For this review, use the dimensioned drawing (mm, ordinates from the lowest corner) and the shaded views. Give positions to 0.01 mm unless a question says otherwise; leave off trailing zeros. Order: outer loops, then holes, each group sorted by start corner. A loop starts at its lowest first (then second) coordinate and runs counter-clockwise, first axis right, second up. Notation, with made-up numbers: (67.5, 54.25) - (101.5, 54.25) arc R17 ccw to (101.5, 76.25) - close; hole circle Ø5 at (47.5, 88.5). An arc over 180 degrees is marked (long way). One line per item, written item: value.
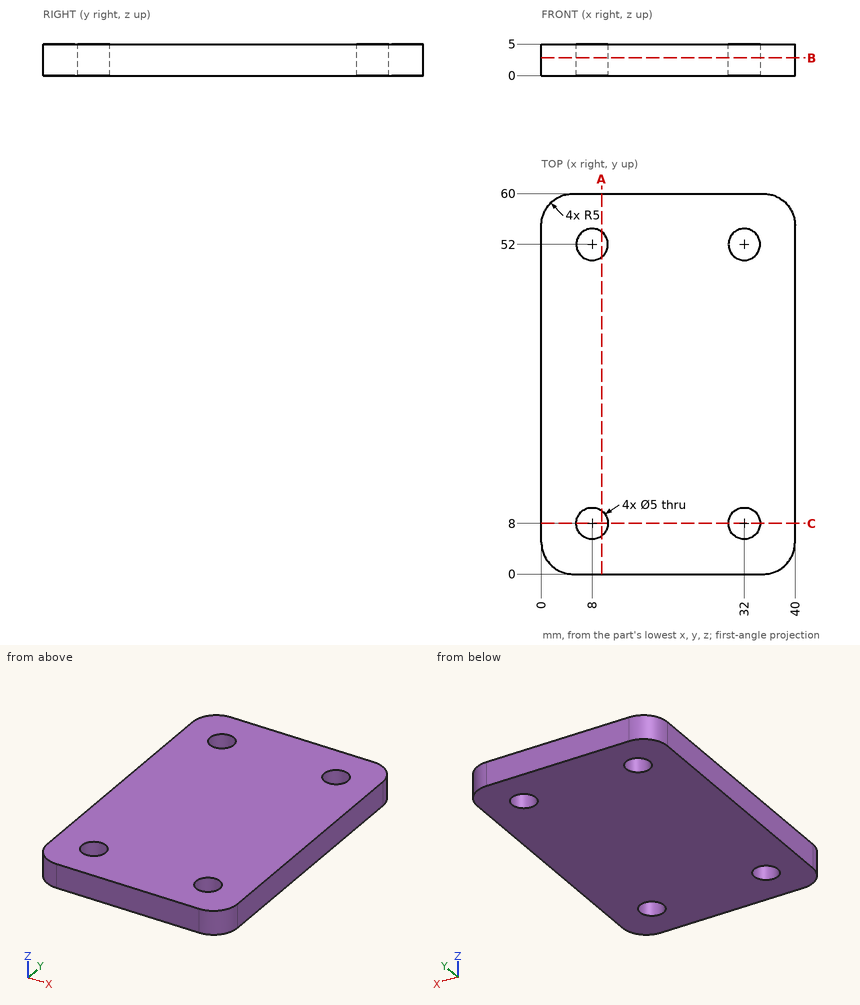
(1) Wall thickness on line 1 (Y direction, x = 32, z = 1.2); line 2 (X direction, y = 8, z = 4); line 3 (Y direction, x = 36, z = 3.95): over which ranges is each line inside the solid? List them lowest first. Write a range as from..to.
Answers below:
line 1: y = 0..5.5, 10.5..49.5, 54.5..60
line 2: x = 0..5.5, 10.5..29.5, 34.5..40
line 3: y = 0.1..59.9
(2) Take a section at B-B (z = 2.8). Write out the cut boundary in (x, y), then the cut area to 3 significant figures.
Answers below:
outline: (0, 5) arc R5 ccw to (5, 0) - (35, 0) arc R5 ccw to (40, 5) - (40, 55) arc R5 ccw to (35, 60) - (5, 60) arc R5 ccw to (0, 55) - close; hole circle Ø5 at (8, 8); hole circle Ø5 at (8, 52); hole circle Ø5 at (32, 8); hole circle Ø5 at (32, 52)
area: 2,300 mm^2
(3) Take a section at C-C (y = 8). Write out the cut boundary in (x, z), then the cut area to 3 significant figures.
Answers below:
outline: (0, 0) - (5.5, 0) - (5.5, 5) - (0, 5) - close; (10.5, 0) - (29.5, 0) - (29.5, 5) - (10.5, 5) - close; (34.5, 0) - (40, 0) - (40, 5) - (34.5, 5) - close
area: 150 mm^2
(4) Take a section at A-A (x = 9.5). Write out the cut boundary in (y, z).
Answers below:
outline: (0, 0) - (6, 0) - (6, 5) - (0, 5) - close; (10, 0) - (50, 0) - (50, 5) - (10, 5) - close; (54, 0) - (60, 0) - (60, 5) - (54, 5) - close
